Source: CAD feature listing. Evaluate the final solid. Frame: model axes, mm. A direction names the side the tool comes from. Round coordinates to 2 decimals unless told otherwise and drop trailing zeros. Loops run counter-clockwise (first coordinate to the right, second up) from the corner with the lowest first, then second, coordinate; pieces in that order, holes last. Notation, with made-up numbers: (66, 40.5) - (73, 40.5) arc R20 ccw to (73, 72.5) - close; hole circle Ø7 at (30, 69.5). An arc over 180 degrees is marked (long way). One line per question, with ' | ' between items. Start each with the question number.
1. Ray query, line 1 (Y direction, x = 9.25, z = -44) (3 decimals); line 2 (Y direction, x = 3, z = -41); line 3 (X direction, y = -12.75, z = -26.5). Return the intervals inside material, ascending.
2. Access query for faces 5 (the flat face through (7.806, -6.392, -25.35)), 6 (the flat face through (-14, 4, -25)), 7 (the flat face through (14, -4, -25)). Directions: +Z, -Z, +X, -X, +Y, -Y. A direction counts if a zero-diameter tool reaches every point of the face in a straight line with its end or side. Return the directions, or none.
3. Cut plane B-B (x = 7). Return loops of the section in (y, z).
4. Pin query (flat end, axial travel): pin 1 (1.6 mm diameter, centred on x = 14, z = -15.5, fed in from +Y); pin 2 (1 mm diameter, centred on x = -11.5, y = 3.5, fed in from +Z); pin 3 (0.6 mm diameter, centred on x = 14.5, z = -22.5, fed in from -Y); pin 4 (2 mm diameter, centred on y = 2.5, z = -29, fed in from +X). Return the tip coordinate at first contact, or that it passes through.
5. Cut plane D-D (x = -10.75). Return loops of the section in (y, z) (3 decimals), then the cut area to 3 significant figures.
6. Mould query, pull axis Y, two halves, no side actions, for faces 1 (the flat face through (-6, 13, -25)), 2 (the flat face through (-8.25, 11, -25)), 3 (the flat face through (4, 0, -50)), 4 (the flat face through (8, 15, -25)). Classes: pulls with the +Y half, pulls with the -Y half, needs draft (parallel to the pull), parting line crosses it, or undercut.
7. Cut plane A-A (y = -11.75). Return loops of the section in (x, z), then the cut area to 3 significant figures.
8. Cut plane C-C (y = 2.75). Return loops of the section in (x, z).
```python
from build123d import *

# Parameters (mm, degrees)
SKETCH1_R      = 3.4
SKETCH1_R_2    = 2.1
EXTRUDE1_DEPTH = 50


with BuildPart() as part:
    # Sketch1 → Extrude1 (new body)
    with BuildSketch(Plane(origin=(0, 0, -50), x_dir=(-1, 0, 0), z_dir=(0, 0, -1))):
        with BuildLine():
            Line((13, 4), (15, 4))
            Line((15, 4), (15, 13))
            ThreePointArc((15, 13), (14.414213562, 14.414213562), (13, 15))
            Line((13, 15), (4, 15))
            Line((4, 15), (4, 13))
            Line((4, 13), (8.25, 13))
            Line((8.25, 13), (8.25, 9.664213562))
            Line((8.25, 9.664213562), (4.585786438, 6))
            Line((4.585786438, 6), (0.519615242, 6))
            Line((0.519615242, 6), (0, 5.7))
            Line((0, 5.7), (-0.519615242, 6))
            Line((-0.519615242, 6), (-4.585786438, 6))
            Line((-4.585786438, 6), (-8.25, 9.664213562))
            Line((-8.25, 9.664213562), (-8.25, 13))
            Line((-8.25, 13), (-4, 13))
            Line((-4, 13), (-4, 15))
            Line((-4, 15), (-13, 15))
            ThreePointArc((-13, 15), (-14.414213562, 14.414213562), (-15, 13))
            Line((-15, 13), (-15, 4))
            Line((-15, 4), (-13, 4))
            Line((-13, 4), (-13, 8.25))
            Line((-13, 8.25), (-9.664213562, 8.25))
            Line((-9.664213562, 8.25), (-6, 4.585786438))
            Line((-6, 4.585786438), (-6, 0.519615242))
            Line((-6, 0.519615242), (-5.7, 0))
            Line((-5.7, 0), (-6, -0.519615242))
            Line((-6, -0.519615242), (-6, -4.585786438))
            Line((-6, -4.585786438), (-9.664213562, -8.25))
            Line((-9.664213562, -8.25), (-13, -8.25))
            Line((-13, -8.25), (-13, -4))
            Line((-13, -4), (-15, -4))
            Line((-15, -4), (-15, -13))
            ThreePointArc((-15, -13), (-14.414213562, -14.414213562), (-13, -15))
            Line((-13, -15), (13, -15))
            ThreePointArc((13, -15), (14.414213562, -14.414213562), (15, -13))
            Line((15, -13), (15, -4))
            Line((15, -4), (13, -4))
            Line((13, -4), (13, -8.25))
            Line((13, -8.25), (9.664213562, -8.25))
            Line((9.664213562, -8.25), (6, -4.585786438))
            Line((6, -4.585786438), (6, -0.519615242))
            Line((6, -0.519615242), (5.7, 0))
            Line((5.7, 0), (6, 0.519615242))
            Line((6, 0.519615242), (6, 4.585786438))
            Line((6, 4.585786438), (9.664213562, 8.25))
            Line((9.664213562, 8.25), (13, 8.25))
            Line((13, 8.25), (13, 4))
        make_face()
        Circle(SKETCH1_R, mode=Mode.SUBTRACT)
        with Locations((-11.625, 11.625)):
            Circle(SKETCH1_R_2, mode=Mode.SUBTRACT)
        with Locations((11.625, 11.625)):
            Circle(SKETCH1_R_2, mode=Mode.SUBTRACT)
        with BuildLine():
            Line((8.701344475, -13), (-8.701344475, -13))
            ThreePointArc((-8.701344475, -13), (-9.142947405, -12.42128559), (-9.817712369, -12.694444444))
            ThreePointArc((-9.817712369, -12.694444444), (-13.44925784, -12.665232346), (-11.625, -9.525))
            Line((-11.625, -9.525), (-8.110786438, -9.525))
            Line((-8.110786438, -9.525), (-4.585786438, -6))
            Line((-4.585786438, -6), (4.585786438, -6))
            Line((4.585786438, -6), (8.110786438, -9.525))
            Line((8.110786438, -9.525), (11.625, -9.525))
            ThreePointArc((11.625, -9.525), (13.44925784, -12.665232346), (9.817712369, -12.694444444))
            ThreePointArc((9.817712369, -12.694444444), (9.142947405, -12.42128559), (8.701344475, -13))
        make_face(mode=Mode.SUBTRACT)
    extrude(amount=-EXTRUDE1_DEPTH)


solid = part.part
```
Answers follow:
1) line 1: y = -15 to -12.402, -9.525 to -7.836, 7.836 to 15 | line 2: y = -15 to -13, -6 to -1.6, 1.6 to 6 | line 3: x = -15 to -13.4, -9.85 to -8.76, 8.76 to 9.85, 13.4 to 15
2) face 5: +Z, -Z | face 6: +Z, -Z, -X | face 7: +Z, -Z, +X
3) outline: (-15, -50) - (-13, -50) - (-13, 0) - (-15, 0) - close; (-8.41, -50) - (-5.59, -50) - (-5.59, 0) - (-8.41, 0) - close; (5.59, -50) - (8.41, -50) - (8.41, 0) - (5.59, 0) - close; (13, -50) - (15, -50) - (15, 0) - (13, 0) - close
4) pin 1: stops at y = 14.99 | pin 2: passes through | pin 3: stops at y = -14.6 | pin 4: stops at x = 6
5) outline: (-15, -50) - (-13.534, -50) - (-13.534, 0) - (-15, 0) - close; (-9.525, -50) - (-8.25, -50) - (-8.25, 0) - (-9.525, 0) - close; (8.25, -50) - (9.716, -50) - (9.716, 0) - (8.25, 0) - close; (13.534, -50) - (15, -50) - (15, 0) - (13.534, 0) - close | area: 284 mm2
6) face 1: undercut | face 2: undercut | face 3: needs draft | face 4: pulls with the +Y half
7) outline: (-15, -50) - (-13.72, -50) - (-13.72, 0) - (-15, 0) - close; (13.72, -50) - (15, -50) - (15, 0) - (13.72, 0) - close | area: 128 mm2
8) outline: (-6, -50) - (-2, -50) - (-2, 0) - (-6, 0) - close; (2, -50) - (6, -50) - (6, 0) - (2, 0) - close
